```python
from build123d import *

# Parameters (mm, degrees)
SKETCH1_W           = 40
SKETCH1_H           = 40
BOSS_EXTRUDE1_DEPTH = 5
SKETCH2_R           = 10
CUT_EXTRUDE1_DEPTH  = 5
SKETCH3_R           = 1.5
CUT_EXTRUDE2_DEPTH  = 5
SKETCH4_R           = 1.5
CUT_EXTRUDE3_DEPTH  = 5


with BuildPart() as part:
    # Sketch1 → Boss-Extrude1 (new body)
    with BuildSketch(Plane.XY):
        Rectangle(SKETCH1_W, SKETCH1_H)
    extrude(amount=BOSS_EXTRUDE1_DEPTH)

    # Sketch2 → Cut-Extrude1 (cut)
    with BuildSketch(Plane(origin=(0, 0, 0), x_dir=(-1, 0, 0), z_dir=(0, 0, -1))):
        Circle(SKETCH2_R)
    extrude(amount=-CUT_EXTRUDE1_DEPTH, mode=Mode.SUBTRACT)

    # Sketch3 → Cut-Extrude2 (cut)
    with BuildSketch(Plane(origin=(0, 0, 0), x_dir=(-1, 0, 0), z_dir=(0, 0, -1))):
        with Locations((0, 15)):
            Circle(SKETCH3_R)
        with Locations((12.990381057, -7.5)):
            Circle(SKETCH3_R)
        with Locations((-12.990381057, -7.5)):
            Circle(SKETCH3_R)
    extrude(amount=-CUT_EXTRUDE2_DEPTH, mode=Mode.SUBTRACT)

    # Sketch4 → Cut-Extrude3 (cut)
    with BuildSketch(Plane(origin=(0, 0, 0), x_dir=(-1, 0, 0), z_dir=(0, 0, -1))):
        with Locations((-17, 17)):
            Circle(SKETCH4_R)
        with Locations(Location((17, 17, 0), (0, 0, 180))):
            Circle(SKETCH4_R)
        with Locations((17, -17)):
            Circle(SKETCH4_R)
        with Locations(Location((-17, -17, 0), (0, 0, 180))):
            Circle(SKETCH4_R)
    extrude(amount=-CUT_EXTRUDE3_DEPTH, mode=Mode.SUBTRACT)


solid = part.part
```
Build history of the part. All positions in model axes, mm. Round coordinates to 2 decimals unless told otherwise and drop trailing zeros. Loops run counter-clockwise (first coordinate to the right, second up) from the corner with the lowest first, then second, coordinate; pieces in that order, holes last. Notation, with made-up numbers: M 32.5,54 L 40.5,54 A22 cw 40.5,73 Z; hole C 12.25,-29.5 d10. An arc over 180 degrees is marked long. Answer as CSV lines item,"result".
1. Flat gauge pin, fed straight in: P1, Ø16, axis at x = 0, y = 0, coming from the +Z side. Where does the tip first touch, or does it go through?
Resolved:
P1,"passes through"
2. Wall check: probe 1 along Y at (x, z) = (-17, 1.5); probe 2 along Y at (x, z) = (0, 2.1); probe 3 along X at (y, z) = (2.5, 3.65). Give the ranges that are in metal, low to high. Write a range as [from, to].
Resolved:
probe 1,"y = [-20, -18.5], [-15.5, 15.5], [18.5, 20]"
probe 2,"y = [-20, -10], [10, 13.5], [16.5, 20]"
probe 3,"x = [-20, -9.68], [9.68, 20]"
3. Cut at A-A on y = -17. Write the cut outline in (x, z).
Resolved:
outline,"M -20,0 L -18.5,0 L -18.5,5 L -20,5 Z; M -15.5,0 L 15.5,0 L 15.5,5 L -15.5,5 Z; M 18.5,0 L 20,0 L 20,5 L 18.5,5 Z"
4. Cut at B-B on y = 0. Write the cut outline in (x, z), then the cut area to 3 significant figures.
Resolved:
outline,"M -20,0 L -10,0 L -10,5 L -20,5 Z; M 10,0 L 20,0 L 20,5 L 10,5 Z"
area,"100 mm²"
5. Two-plate mould, pull along X, no slides. Class faces 1 (the flat face through (20, 0, 2)), 2 (the flat face through (-5, 9, 5)), 3 (the cylindrical face through (-18.5, 16.93, 2.46)): released by +X, released by -X, zero draft, split by the parting line, or undercut.
Resolved:
face 1,"released by +X"
face 2,"zero draft"
face 3,"undercut"
6. Cut at D-D on z = 0.7. Count the separate pieces of the cut face and the enclosed holes in it, then the cut area to 3 significant figures.
Resolved:
separate pieces,"1"
enclosed holes,"8"
area,"1,240 mm²"
7. Cut at C-C on x = 0. Write the cut outline in (y, z).
Resolved:
outline,"M -20,0 L -10,0 L -10,5 L -20,5 Z; M 10,0 L 13.5,0 L 13.5,5 L 10,5 Z; M 16.5,0 L 20,0 L 20,5 L 16.5,5 Z"
